Part model, mm, in its own coordinate system. A direction names the side the tool comes from. Coordinates: 2 decimals unless noted, no trailing zeros. Loops run counter-clockwise (first coordinate to the right, second up) from the corner with the lowest first, then second, coordinate; pieces in that order, holes last. Notation, with made-up numbers: (30, 4.25) -> (89, 4.25) arc R4 cw to (89, 8.25) -> close; hole circle Ø5 at (43, 13.5). An arc over 180 degrees is marked (long way). Use one line per item in the form item = value. Start each with the question number.
(1) Pin check, flat tips, straight feed: P1, Ø1, axis at y = -9, z = -8.5, coming from the -X side; P2, Ø2.5, axis at y = 9, z = 10.5, coming from the -X side. Stop position of each tip, or through.
(2) Band-saw the part on C-C on x = 4.25. Count the separate pieces of the cut face and the enclosed holes in it, then the cut area to 3 significant figures.
(3) Drill centre lines: L1, parallel to Y at x = 3.85, z = 11.8; L2, parallel to Y at x = 4.7, z = -8.5; L3, parallel to Y at x = 1.55, z = 12.5. Where is each one in solid material? Low to high. Write a range as [from, to].
(4) 3-axis set-ups, long thin cutter, end or side, ignore diameter. For faces 1 (the cylindrical face through (1.78, -0.61, 6.68)), 2 (the cylindrical face through (4.51, 9.99, -8.37)): which of +Z, -Z, +X, -X, +Y, -Y reach the whole face in a straight line?
(5) Mould opens along Z. For faces 3 (the cylindrical face through (2.736, -12.899, -13.715)), 4 (the cylindrical face through (1.78, 7.44, -8.85)), 5 (the flat face through (0, 0, 3)), 6 (the cylindrical face through (4.51, 9.99, 10.63)) say: +Z half, -Z half, draft (parallel to the pull), parting line (faces both ways), or undercut.
(6) Band-saw the part on A-A on z = -0.4. Give the cut face in (x, y), then the cut area to 3 significant figures.
(7) Band-saw the part on B-B on y = -6. Give the cut face in (x, z).
```python
from build123d import *

# Parameters (mm, degrees)
SKETCH_1_W                    = 26.4
SKETCH_1_H                    = 28
EXTRUDE_1_DEPTH               = 5.5
HOLE_WIZARD_1_6_1_6_1_D       = 1.6
HOLE_WIZARD_2_5_2_5_1_D       = 2.5
HOLE_WIZARD_1_6_1_6_2_D       = 1.6
HOLE_WIZARD_2_5_2_5_2_D       = 2.5
HOLE_WIZARD_5_0_5_1_D         = 5
HOLE_WIZARD_M1_61_D           = 2
HOLE_WIZARD_M1_61_CBORE_D     = 3.2
HOLE_WIZARD_M1_61_CBORE_DEPTH = 3.5
FILLET_1_R                    = 1
CHAMFER_1_SIZE2               = 0.6
CHAMFER_1_SIZE                = 0.599999999
CHAMFER_2_SIZE                = 0.1
CHAMFER_3_SIZE                = 0.2


with BuildPart() as part:
    # Эскиз1 → Бобышка-Вытянуть1 (new body)
    with BuildSketch(Plane(origin=(0, 0, 0), x_dir=(0, -1, 0), z_dir=(-1, 0, 0))):
        Rectangle(SKETCH_1_W, SKETCH_1_H)
    extrude(amount=-EXTRUDE_1_DEPTH)

    # Диаметр отверстия Ø1.6 (1.6)1 (through all)
    with Locations(Plane.ZY):
        with Locations((-10.2, -6), (11.8, -6), (11.8, 6)):
            Hole(HOLE_WIZARD_1_6_1_6_1_D / 2)

    # Диаметр отверстия Ø2.5 (2.5)1 (through all)
    with Locations(Plane(origin=(5.5, 0, 0), x_dir=(0, 0, -1), z_dir=(1, 0, 0))):
        with Locations((11.8, -10)):
            Hole(HOLE_WIZARD_2_5_2_5_1_D / 2)

    # Диаметр отверстия Ø1.6 (1.6)2 (through all)
    with Locations(Plane(origin=(5.5, 0, 0), x_dir=(0, 0, -1), z_dir=(1, 0, 0))):
        with Locations((10.2, 6)):
            Hole(HOLE_WIZARD_1_6_1_6_2_D / 2)

    # Диаметр отверстия Ø2.5 (2.5)2 (through all)
    with Locations(Plane.ZY):
        with Locations((-11.8, 10), (11.8, 0)):
            Hole(HOLE_WIZARD_2_5_2_5_2_D / 2)

    # Диаметр отверстия Ø5.0 (5)1 (through all)
    with Locations(Plane(origin=(5.5, 0, 0), x_dir=(0, 0, -1), z_dir=(1, 0, 0))):
        with Locations((0.4, 0)):
            Hole(HOLE_WIZARD_5_0_5_1_D / 2)

    # Цековка для винта с внутренним шестигранником M1.61 (through all)
    with Locations(Plane.ZY):
        with Locations((-8.5, 9), (-8.5, -9), (5.2, 0), (10.5, -9), (10.5, 9)):
            CounterBoreHole(HOLE_WIZARD_M1_61_D / 2, HOLE_WIZARD_M1_61_CBORE_D / 2, HOLE_WIZARD_M1_61_CBORE_DEPTH)

    # Скругление1
    fillet_1_edges = [part.edges().sort_by_distance(p)[0] for p in [
        (2.75, -13.2, 14),
        (2.75, -13.2, -14),
        (2.75, 13.2, -14),
        (2.75, 13.2, 14),
    ]]
    fillet(fillet_1_edges, radius=FILLET_1_R)

    # Фаска1
    chamfer_1_edges = [part.edges().sort_by_distance(p)[0] for p in [
        (5.5, 0, -2.9),
        (0, 0, -2.9),
    ]]
    chamfer(chamfer_1_edges, length=CHAMFER_1_SIZE, length2=CHAMFER_1_SIZE2)

    # Фаска2
    chamfer_2_edges = [part.edges().sort_by_distance(p)[0] for p in [
        (0, 6, 12.6),
        (5.5, 6, 12.6),
        (0, -6, 12.6),
        (5.5, -6, 12.6),
        (0, -6, -9.4),
        (5.5, -6, -9.4),
        (5.5, -10, -13.05),
        (0, -10, -13.05),
        (5.5, 6, -11),
        (0, 6, -11),
        (0, 0, 13.05),
        (5.5, 0, 13.05),
        (0, 10, -10.55),
        (5.5, 10, -10.55),
        (0, 9, 8.9),
        (5.5, 9, 11.5),
        (3.5, 9, 11.5),
        (0, -9, 8.9),
        (5.5, -9, 11.5),
        (3.5, -9, 11.5),
        (0, 0, 3.6),
        (5.5, 0, 6.2),
        (3.5, 0, 6.2),
        (0, -9, -10.1),
        (5.5, -9, -7.5),
        (3.5, -9, -7.5),
        (0, 9, -10.1),
        (5.5, 9, -7.5),
        (3.5, 9, -7.5),
        (0, 0, 14),
        (0, 13.2, 0),
        (0, 0, -14),
        (0, -13.2, 0),
        (0, -12.907106781, 13.707106781),
        (0, -12.907106781, -13.707106781),
        (0, 12.907106781, -13.707106781),
        (0, 12.907106781, 13.707106781),
    ]]
    chamfer(chamfer_2_edges, length=CHAMFER_2_SIZE)

    # Фаска3
    chamfer_3_edges = [part.edges().sort_by_distance(p)[0] for p in [
        (5.5, 0, 14),
        (5.5, 13.2, 0),
        (5.5, -13.2, 0),
        (5.5, 0, -14),
        (5.5, -12.907106781, 13.707106781),
        (5.5, -12.907106781, -13.707106781),
        (5.5, 12.907106781, -13.707106781),
        (5.5, 12.907106781, 13.707106781),
    ]]
    chamfer(chamfer_3_edges, length=CHAMFER_3_SIZE)


solid = part.part
```
A:
q1.P1 = through
q1.P2 = 3.5
q2.separate_pieces = 1
q2.enclosed_holes = 13
q2.area = 680 mm²
q3.L1 = [-13.2, -6.8], [-5.2, -1.25], [1.25, 5.2], [6.8, 13.2]
q3.L2 = [-13.2, -10], [-8, 8], [10, 13.2]
q3.L3 = [-13.2, -6.39], [-5.61, -1.04], [1.04, 5.61], [6.39, 13.2]
q4.face_1 = -X
q4.face_2 = +X, -X
q5.face_3 = -Z half
q5.face_4 = undercut
q5.face_5 = draft
q5.face_6 = undercut
q6.outline = (0, -13.1) -> (0.1, -13.2) -> (5.3, -13.2) -> (5.5, -13) -> (5.5, -3.1) -> (4.9, -2.5) -> (0.6, -2.5) -> (0, -3.1) -> close; (0, 3.1) -> (0.6, 2.5) -> (4.9, 2.5) -> (5.5, 3.1) -> (5.5, 13) -> (5.3, 13.2) -> (0.1, 13.2) -> (0, 13.1) -> close
q6.area = 117 mm²
q7.outline = (0, -13.9) -> (0.1, -14) -> (5.3, -14) -> (5.5, -13.8) -> (5.5, -11.1) -> (5.4, -11) -> (0.1, -11) -> (0, -11.1) -> close; (0, -9.3) -> (0.1, -9.4) -> (5.4, -9.4) -> (5.5, -9.3) -> (5.5, 10.9) -> (5.4, 11) -> (0.1, 11) -> (0, 10.9) -> close; (0, 12.7) -> (0.1, 12.6) -> (5.4, 12.6) -> (5.5, 12.7) -> (5.5, 13.8) -> (5.3, 14) -> (0.1, 14) -> (0, 13.9) -> close
